The model under review builds one solid part; all positions refer to its coordinate system, in mm. A direction names the side the tool comes from. Give positions to 0.01 mm unless a question says otherwise; leave off trailing zeros. Order: outer loops, then holes, each group sorted by start corner. A loop starts at its lowest first (then second) coordinate and runs counter-clockwise, first axis right, second up.
```python
from build123d import *

# Parameters (mm, degrees)
F0_R     = 12.7
F1_DEPTH = 25.4
F2_R     = 5.754427
F4_DEPTH = 25.4
F3_R     = 5.992973
F5_DEPTH = 25.4


with BuildPart() as f1:
    # F0 (on Front) → F1 (new body)
    with BuildSketch(Plane.XZ):
        with BuildLine():
            Line((-33.539512, -9.618156), (-62.502647, -9.618156))
            Line((-62.502647, -9.618156), (-62.502647, -22.318156))
            Line((-62.502647, -22.318156), (64.497353, -22.318156))
            Line((64.497353, -22.318156), (64.497353, -9.618156))
            Line((64.497353, -9.618156), (28.306579, -9.618156))
            ThreePointArc((28.306579, -9.618156), (19.970903, -6.499727), (15.728804, 1.324127))
            ThreePointArc((15.728804, 1.324127), (-2.616467, 18.350258), (-20.961737, 1.324127))
            ThreePointArc((-20.961737, 1.324127), (-25.203836, -6.499727), (-33.539512, -9.618156))
        make_face()
        with Locations((-4.936342, 3.67939)):
            Circle(F0_R, mode=Mode.SUBTRACT)
    extrude(amount=F1_DEPTH)

    # F2 (on face) → F4 (cut)
    with BuildSketch(Plane.XY.offset(-9.618156)):
        with Locations((-44.681605, -12.206142)):
            Circle(F2_R)
    extrude(amount=-F4_DEPTH, mode=Mode.SUBTRACT)

    # F3 (on face) → F5 (cut)
    with BuildSketch(Plane.XY.offset(-9.618156)):
        with Locations((45.22102, -13.935037)):
            Circle(F3_R)
    extrude(amount=-F5_DEPTH, mode=Mode.SUBTRACT)


solid = f1.part
```
Item 1: For line 1 (X direction, y = -14.25, z = -19.5); line 2 (Z direction, x = 0, y = -19); line 3 (Z direction, x = 56, y = -5), list the stretches that pass through material, from the lowest coordinate up.
Values found:
line 1: x = -62.5 to -50.06, -39.3 to 39.24, 51.21 to 64.5
line 2: z = -22.32 to -8.02, 15.38 to 18.16
line 3: z = -22.32 to -9.62
Item 2: Draft analysis for pull direction Y (two halves, no side actions). For faces 1 (the flat face through (0, 0, -11)), 2 (the cylindrical face through (-39.193, -10.478, -15.879)), 3 (the flat face through (-62.503, -13, -16)), 4 (the cylindrical face through (39.234, -13.672, -15.879)), state which applies: released by +Y, released by -Y, zero draft, split by the parting line, or undercut.
Values found:
face 1: released by +Y
face 2: undercut
face 3: zero draft
face 4: undercut
Item 3: Take a section at A-A (z = -0.5). Give the boundary of the cut face in (x, y).
Values found:
outline: (-21.36, -25.4) - (-16.93, -25.4) - (-16.93, 0) - (-21.36, 0) - close; (7.06, -25.4) - (16.12, -25.4) - (16.12, 0) - (7.06, 0) - close
Item 4: Take a section at B-B (x = 6.5). Give the boundary of the cut face in (y, z), and give its area (3 significant figures).
Values found:
outline: (-25.4, -22.32) - (0, -22.32) - (0, -1.84) - (-25.4, -1.84) - close; (-25.4, 9.2) - (0, 9.2) - (0, 15.93) - (-25.4, 15.93) - close
area: 691 mm2
Item 5: Take a section at C-C (y = -4.75). Give the boundary of the cut face in (x, z).
Values found:
outline: (-62.5, -22.32) - (64.5, -22.32) - (64.5, -9.62) - (28.31, -9.62) arc R12.7 cw to (15.73, 1.32) arc R18.4 ccw to (-20.96, 1.32) arc R12.7 cw to (-33.54, -9.62) - (-62.5, -9.62) - close; hole circle Ø25.4 at (-4.94, 3.68)
Item 6: Clearance check with flat-ended pins moving along their axes: pin 1 Ø12 at (y, z) = (-3.5, -4) entering from +X; pin 2 Ø23 at (x, z) = (-4.94, 3.68) entering from +Y; pin 3 Ø2 at (y, z) = (-6, 8) entering from -X; pin 4 Ø10 at (y, z) = (-7.5, 10) entering from -X. State where each tip first meets the part, or that it passes through.
Values found:
pin 1: stops at x = 64.5
pin 2: passes through
pin 3: stops at x = -19.61
pin 4: stops at x = -20.31
Item 7: For faces 5 (the flat face through (-51, -13, -9.618)), 6 (the flat face through (51, -10, -9.618)), 7 (the cylindrical face through (-14.3, -12.52, 12.26)), list the 3-axis set-ups (+Z, -Z, +X, -X, +Y, -Y) from which the entire face can be reached by the end or side of a thin tool; tool diameter is ignored.
Values found:
face 5: +Z, -X, +Y, -Y
face 6: +Z, +X, +Y, -Y
face 7: +Y, -Y
Item 8: Take a section at D-D (x = 32.5). Give the boundary of the cut face in (y, z).
Values found:
outline: (-25.4, -22.32) - (0, -22.32) - (0, -9.62) - (-25.4, -9.62) - close
